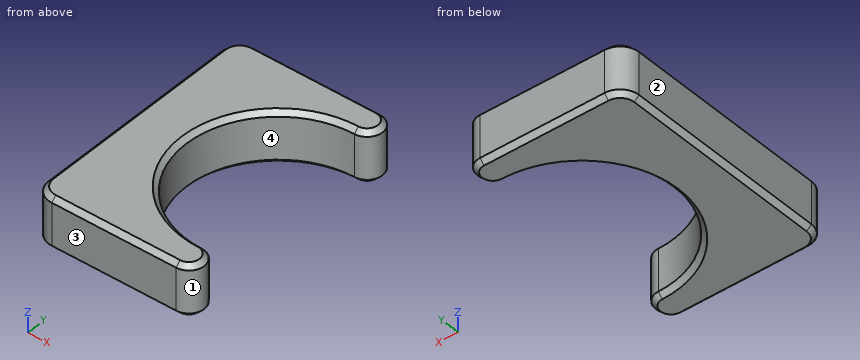
from build123d import *

# Parameters (mm, degrees)
F1_DEPTH = 11
F2_SIZE  = 1


with BuildPart() as f1:
    # F0 (on Top) → F1 (new body)
    with BuildSketch(Plane.XY):
        with BuildLine():
            ThreePointArc((25, -19.5), (5.5, 0), (25, 19.5))
            ThreePointArc((25, 19.5), (28.25, 22.75), (25, 26))
            Line((25, 26), (-1.5, 26))
            ThreePointArc((-1.5, 26), (-4.328427, 24.828427), (-5.5, 22))
            Line((-5.5, 22), (-5.5, -22))
            ThreePointArc((-5.5, -22), (-4.328427, -24.828427), (-1.5, -26))
            Line((-1.5, -26), (25, -26))
            ThreePointArc((25, -26), (28.25, -22.75), (25, -19.5))
        make_face()
    extrude(amount=F1_DEPTH)

    # F2
    f2_edges = [f1.edges().sort_by_distance(p)[0] for p in [
        (5.5, 0, 11),
        (5.5, 0, 0),
    ]]
    chamfer(f2_edges, length=F2_SIZE)


solid = f1.part
Source: CAD feature listing. Evaluate the final solid. Frame: model axes, mm. Face numbers are marked on the shaded views. Give positions to 0.01 mm unless a question says otherwise; leave off trailing zeros. Write each loop counter-clockwise with the first axis right and the second up, starting at its lowest first coordinate (ties: lowest second). Pieces come first, ordered by that corner, then holes. Notation, with made-up numbers: M -18.5,40 L -7.5,40 A34 cw -7.5,75 Z; hole C -10.5,20.5 d2. An arc over 180 degrees is marked long. Return JSON: item names as keys, results as strings. Group by question number.
1) Pull-direction query (Y, two-part tool) for the marked faces 1, 2, 3 and 4; classes: pulls with the +Y half, pulls with the -Y half, needs draft (parallel to the pull), parting line crosses it, or undercut.
2) Pin query (flat end, axial travel): P1, Ø6, axis at y = 14, z = 3, coming from the +X side; P2, Ø5, axis at x = 11.5, y = -8.5, coming from the -Z side. Return the tip coordinate at first contact, or that it passes through.
3) Material intervals for line 1 along Y through (x, z) = (25, 6.75); line 2 along Y through (x, z) = (14, 10.25); line 3 along X through (y, z) = (-7, 8), sorted ascending. Write a range as [from, to].
4) Cut plane A-A, the plane z = 9.25. Output: boundary loops of the cut face in (x, y).
Recorded:
{
 "1": {"face 1": "undercut", "face 2": "needs draft", "face 3": "pulls with the -Y half", "face 4": "undercut"},
 "2": {"P1": "stops at x = 15.45", "P2": "passes through"},
 "3": {"line 1": "y = [-26, -19.5], [19.5, 26]", "line 2": "y = [-25.75, -16.4], [16.4, 25.75]", "line 3": "x = [-5.5, 6.8]"},
 "4": {"outline": "M -5.5,-22 A4 ccw -1.5,-26 L 25,-26 A3.25 ccw 25,-19.5 A19.5 cw 25,19.5 A3.25 ccw 25,26 L -1.5,26 A4 ccw -5.5,22 Z"}
}
